```python
from build123d import *

# Parameters (mm, degrees)
F0_R          = 55.519011
F0_R_2        = 43.738793
F1_DEPTH      = 101.346
F2_W          = 238.856115
F2_H          = 85.85909
F3_DEPTH      = 2.54
F3_DEPTH_BACK = 2.54


with BuildPart() as f1:
    # F0 (on Top) → F1 (new body)
    with BuildSketch(Plane.XY):
        Circle(F0_R)
        Circle(F0_R_2, mode=Mode.SUBTRACT)
    extrude(amount=-F1_DEPTH)

    # F2 (on Front) → F3 (join, two sides)
    with BuildSketch(Plane.XZ) as f3_sk:
        with Locations((5.983558, -107.62085)):
            Rectangle(F2_W, F2_H)
    extrude(amount=F3_DEPTH)
    extrude(f3_sk.sketch, amount=-F3_DEPTH_BACK)


solid = f1.part
```
Check sheet for the modelled part. Datum: model origin and axes. Units: mm. A direction names the side the tool comes from. Round coordinates to 2 decimals unless told otherwise and drop trailing zeros. Order: outer loops, then holes, each group sorted by start corner. A loop starts at its lowest first (then second) coordinate and runs counter-clockwise, first axis right, second up.
1) Mould release check, pull along X, two halves, no side actions. Record for faces 1 (the cylindrical face through (51.285, -21.264, -49.964)), 2 (the flat face through (4, -2.54, -107)), 3 (the flat face through (-4, -45, -101.346)): +X half, -X half, draft (parallel to the pull), parting line (faces both ways), or undercut.
2) Section check B-B (y = 22). Record the boundary of the cut face in (x, z).
3) Section check A-A (x = 0). Record the boundary of the cut face in (y, z).
4) Go/stop test with flat-tipped pins: pin 1 Ø12 at (x, z) = (101, -69) entering from +Y; pin 2 Ø5.5 at (x, y) = (16.5, 1) entering from +Z; pin 3 Ø16 at (x, y) = (12.5, -38.5) entering from -Z. Record where each tip stops, or that it passes through.
5) Scan lines: line 1 (Y direction, x = 0, z = -74); line 2 (Y direction, x = 0, z = -63); line 3 (Y direction, x = 86.5, z = -100.5). Record each from-to range of solid material in increasing order.
6) Tool access check on faces 4 (the flat face through (4, 45, -101.346)), 5 (the flat face through (-85, 0, -64.691)), 6 (the flat face through (90, 0, -64.691)), 7 (the flat face through (-113.444, 0, -108)), 8 (the flat face through (-1, 0, -64.691)). Record the directions out of +Z, -Z, +X, -X, +Y, -Y that give a thin tool (end or side, any length) a straight path to the whole face; none if there is none.
7) Section check D-D (z = -106.5). Record the boundary of the cut face in (x, y), and give its area (3 significant figures).
8) Section check C-C (y = 0). Record the boundary of the cut face in (x, z).
Result:
1. face 1: parting line
1. face 2: undercut
1. face 3: draft
2. outline: (-50.97, -101.35) - (-37.8, -101.35) - (-37.8, 0) - (-50.97, 0) - close; (37.8, -101.35) - (50.97, -101.35) - (50.97, 0) - (37.8, 0) - close
3. outline: (-55.52, -101.35) - (-43.74, -101.35) - (-43.74, 0) - (-55.52, 0) - close; (-2.54, -150.55) - (2.54, -150.55) - (2.54, -64.69) - (-2.54, -64.69) - close; (43.74, -101.35) - (55.52, -101.35) - (55.52, 0) - (43.74, 0) - close
4. pin 1: stops at y = 2.54
4. pin 2: stops at z = -64.69
4. pin 3: stops at z = -101.35
5. line 1: y = -55.52 to -43.74, -2.54 to 2.54, 43.74 to 55.52
5. line 2: y = -55.52 to -43.74, 43.74 to 55.52
5. line 3: y = -2.54 to 2.54
6. face 4: -Z, +X, -X, +Y
6. face 5: +Z, -X, +Y, -Y
6. face 6: +Z, +X, +Y, -Y
6. face 7: +Z, -Z, -X, +Y, -Y
6. face 8: +Z
7. outline: (-113.44, -2.54) - (125.41, -2.54) - (125.41, 2.54) - (-113.44, 2.54) - close
7. area: 1,210 mm2
8. outline: (-113.44, -150.55) - (125.41, -150.55) - (125.41, -64.69) - (55.52, -64.69) - (55.52, 0) - (43.74, 0) - (43.74, -64.69) - (-43.74, -64.69) - (-43.74, 0) - (-55.52, 0) - (-55.52, -64.69) - (-113.44, -64.69) - close
